from build123d import *

# Parameters (mm, degrees)
SKETCH1_R           = 30
BOSS_EXTRUDE1_DEPTH = 75
SKETCH2_R           = 15
BOSS_EXTRUDE2_DEPTH = 35
CUT_EXTRUDE1_REACH  = 82
SKETCH3_W           = 8
SKETCH3_H           = 45


with BuildPart() as part:
    # Sketch1 → Boss-Extrude1 (new body)
    with BuildSketch(Plane.XY):
        Circle(SKETCH1_R)
    extrude(amount=BOSS_EXTRUDE1_DEPTH)

    # Sketch2 → Boss-Extrude2 (add)
    with BuildSketch(Plane.XY.offset(75)):
        with BuildLine():
            Line((-40, 102.46950766), (-40, -102.46950766))
            ThreePointArc((-40, -102.46950766), (0, -110), (40, -102.46950766))
            Line((40, -102.46950766), (40, 102.46950766))
            ThreePointArc((40, 102.46950766), (0, 110), (-40, 102.46950766))
        make_face()
        with Locations((0, -75)):
            Circle(SKETCH2_R, mode=Mode.SUBTRACT)
        with Locations((0, 75)):
            Circle(SKETCH2_R, mode=Mode.SUBTRACT)
    extrude(amount=BOSS_EXTRUDE2_DEPTH)

    # Sketch3 → Cut-Extrude1 (cut, up to next)
    with BuildSketch(Plane(origin=(40, 0, 0), x_dir=(0, 0, -1), z_dir=(1, 0, 0)), mode=Mode.PRIVATE) as cut_extrude1_sk1:
        with Locations((-106, 0)):
            Rectangle(SKETCH3_W, SKETCH3_H)
    cut_extrude1_tool1 = extrude(cut_extrude1_sk1.sketch, amount=-CUT_EXTRUDE1_REACH, mode=Mode.PRIVATE) & part.part
    add(cut_extrude1_tool1.solids().sort_by_distance((40, 0, 106))[0], mode=Mode.SUBTRACT)


solid = part.part
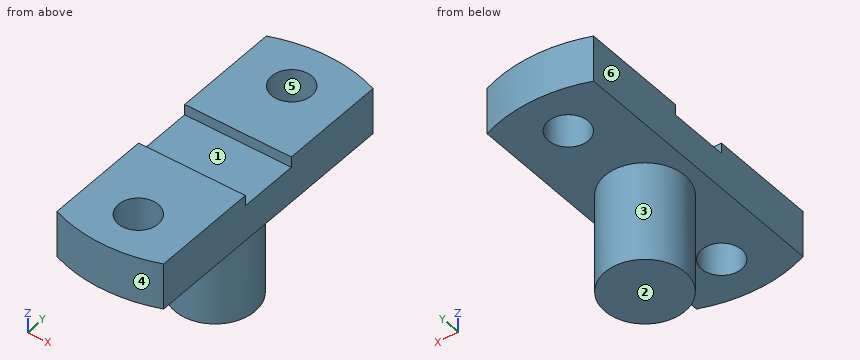
Could you check a few things on this model? Use its own coordinates, in mm. Face numbers are marked on the shaded views. A direction names the side the tool comes from. Give positions to 0.01 mm unless a question says otherwise; leave off trailing zeros. Order: outer loops, then holes, each group sorted by start corner. A loop starts at its lowest first (then second) coordinate and runs counter-clockwise, first axis right, second up. Notation, with made-up numbers: (-26.5, 17) - (-21.5, 17) arc R21 ccw to (-21.5, 42) - close; hole circle Ø10 at (50, 44). An arc over 180 degrees is marked (long way). One line per item, written item: value. Start each with the question number.
1. If I drill on probe 1 along Y at (x, z) = (0, 93.5); probe 2 along Y at (x, z) = (-8.5, 93); probe 3 along Z at (x, y) = (20, 68.5), over which ranges is the centre line in solid material (lowest first)?
2. For P1, Ø12, axis at x = -31, z = 82, coming from the -Y side; P2, Ø4, axis at x = 3.5, z = 104.5, coming from the -Y side; P3, Ø1.5, axis at x = -24, z = 23.5, coming from the -Y side, each with a flat end and sliding along its axis, tell me the tip position at first contact or that it passes through.
3. Imagine slicing it at A-A on y = 75. List the corners of the cut face in (x, z) for me.
4. Imagine slicing it at D-D on x = 17.5. List the corners of the cut face in (y, z) for me.
5. Imagine slicing it at C-C on y = 0. List the corners of the cut face in (x, z) for me, plus the area to 3 significant figures.
6. For the marked faces 1, 2 and 3, which set-ups out of +Z, -Z, +X, -X, +Y, -Y let a thin tool reach every point of the face, with its end or its side?
7. Thinking about a two-plate mould opening in Y: for the marked faces 4, 5 and 6, which applies, +Y half, -Y half, draft (parallel to the pull), parting line (faces both ways), or undercut?
8. Imagine slicing it at B-B on x = 0. List the corners of the cut face in (y, z) for me.
Values:
1. probe 1: -110 to -90, -60 to 60, 90 to 110
1. probe 2: -109.67 to -87.36, -62.64 to 62.64, 87.36 to 109.67
1. probe 3: 75 to 110
2. P1: y = -107.12
2. P2: y = -109.99
2. P3: y = -18.96
3. outline: (-40, 75) - (-15, 75) - (-15, 110) - (-40, 110) - close; (15, 75) - (40, 75) - (40, 110) - (15, 110) - close
4. outline: (-108.6, 75) - (-24.37, 75) - (-24.37, 0) - (24.37, 0) - (24.37, 75) - (108.6, 75) - (108.6, 110) - (22.5, 110) - (22.5, 102) - (-22.5, 102) - (-22.5, 110) - (-108.6, 110) - close
5. outline: (-40, 75) - (-30, 75) - (-30, 0) - (30, 0) - (30, 75) - (40, 75) - (40, 102) - (-40, 102) - close
5. area: 6,660 mm²
6. face 1: +Z, +X, -X
6. face 2: -Z, +X, -X, +Y, -Y
6. face 3: -Z
7. face 4: -Y half
7. face 5: undercut
7. face 6: draft
8. outline: (-110, 75) - (-90, 75) - (-90, 110) - (-110, 110) - close; (-60, 75) - (-30, 75) - (-30, 0) - (30, 0) - (30, 75) - (60, 75) - (60, 110) - (22.5, 110) - (22.5, 102) - (-22.5, 102) - (-22.5, 110) - (-60, 110) - close; (90, 75) - (110, 75) - (110, 110) - (90, 110) - close
